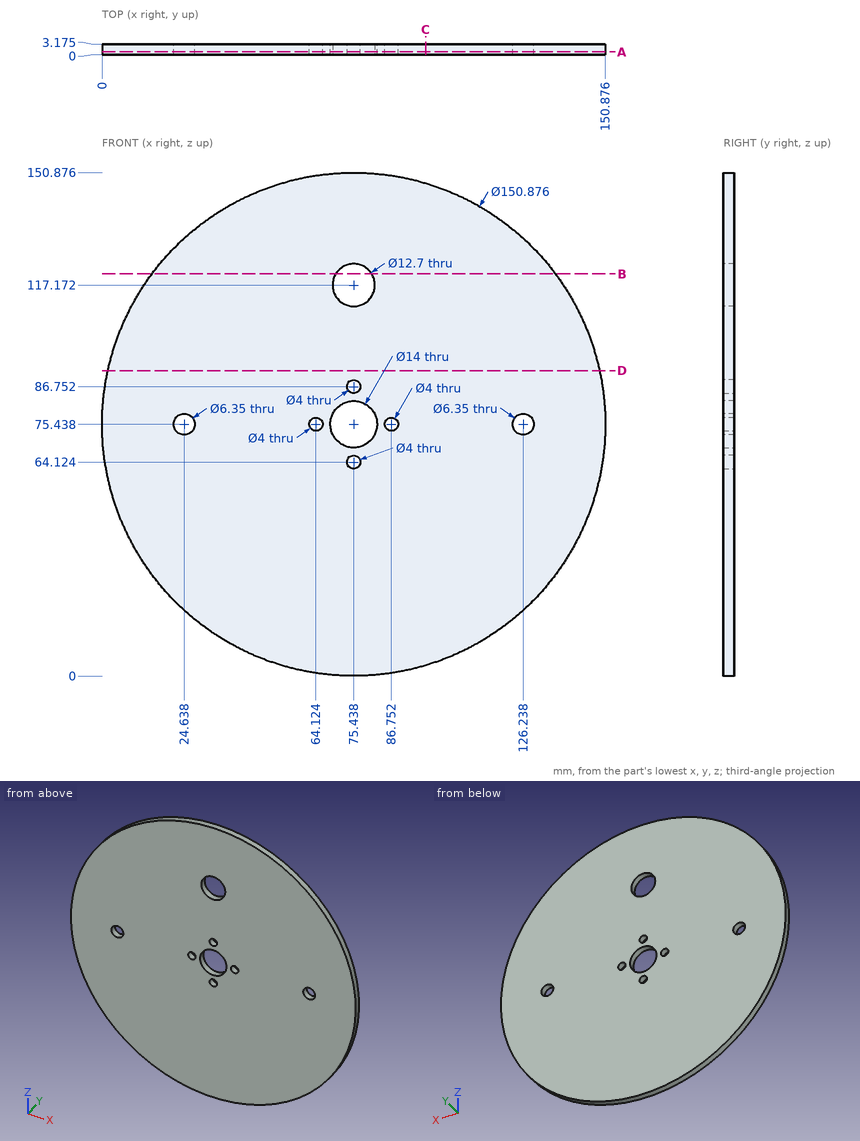
Geometry check sheet. Reference: drawing and pictorial views, mm from the part's lowest x, y, z. Round coordinates to 2 decimals unless told otherwise and drop trailing zeros. Loops run counter-clockwise (first coordinate to the right, second up) from the corner with the lowest first, then second, coordinate; pieces in that order, holes last. Notation, with made-up numbers: (87, 45.5) -> (95, 45.5) arc R25 ccw to (95, 65.5) -> close; hole circle Ø6 at (78, 72). An arc over 180 degrees is marked (long way). Use a Markdown table: item, result.
(1) Scan lines: probe 1 along Z at (x, y) = (71, 1.3) (1 decimal); probe 2 along X at (y, z) = (0.2, 86.5) (1 decimal); probe 3 along X at (y, z) = (0.6, 88.5) (1 decimal). Record each from-to range of solid material in increasing order.
Calculated:
| item | result |
|---|---|
| probe 1 | 0.1 to 70, 80.9 to 112.6, 121.7 to 150.7 |
| probe 2 | 0.8 to 73.5, 77.4 to 150.1 |
| probe 3 | 1.1 to 74.5, 76.4 to 149.7 |
(2) Sectioned sample at D-D (z = 91.5). Enter the section's corners in (x, y) (1 decimal).
Calculated:
| item | result |
|---|---|
| outline | (1.7, 0) -> (149.1, 0) -> (149.1, 3.2) -> (1.7, 3.2) -> close |
(3) Sectioned sample at B-B (z = 120.5). Enter the section's corners in (x, y) (1 decimal), then the cut area to 3 significant figures.
Calculated:
| item | result |
|---|---|
| outline | (14.9, 0) -> (70, 0) -> (70, 3.2) -> (14.9, 3.2) -> close; (80.8, 0) -> (135.9, 0) -> (135.9, 3.2) -> (80.8, 3.2) -> close |
| area | 350 mm² |
(4) Sectioned sample at C-C (x = 97). Enter the section's corners in (y, z) (3 decimals).
Calculated:
| item | result |
|---|---|
| outline | (0, 3.147) -> (3.175, 3.147) -> (3.175, 147.729) -> (0, 147.729) -> close |
(5) Go/stop test with flat-tipped pins: P1, Ø3, axis at x = 75.438, z = 64.124, coming from the +Y side; P2, Ø1.5, axis at y = 0.5, z = 94.5, coming from the -X side. Record where each tip stops, or that it passes through.
Calculated:
| item | result |
|---|---|
| P1 | through |
| P2 | x = 2.26 |
(6) Sectioned sample at A-A (y = 0.8). Give the number of separate pieces and of enclosed holes in the cut face, then the cut area to 3 significant figures.
Calculated:
| item | result |
|---|---|
| separate pieces | 1 |
| enclosed holes | 8 |
| area | 17,500 mm² |
